Design review of the part built by this model. Coordinates are the model's own, in mm. Face numbers are marked on the shaded views. A direction names the side the tool comes from. Coordinates: 2 decimals unless noted, no trailing zeros. Write each loop counter-clockwise with the first axis right and the second up, starting at its lowest first coordinate (ties: lowest second). Pieces come first, ordered by that corner, then holes. Notation, with made-up numbers: (4, 73) - (62, 73) arc R23 ccw to (62, 105) - close; hole circle Ø7 at (62.5, 37). An arc over 180 degrees is marked (long way). Use a Markdown table: item, result.
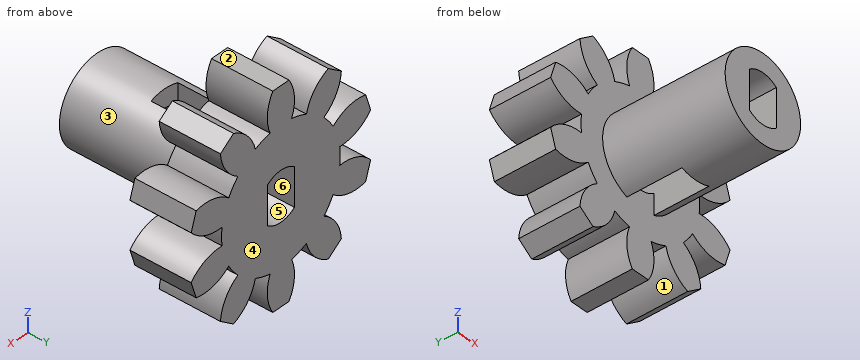
from build123d import *

# Parameters (mm, degrees)
SKETCH_1_R                      = 5.5
EXTRUDE_1_DEPTH                 = 5
EXTRUDE_START                   = -5
EXTRUDE_2_DEPTH                 = 5
SKETCH_3_R                      = 3.5
EXTRUDE_3_DEPTH                 = 10
CUT_EXTRUDE_1_DEPTH             = 20.141619155
CUT_EXTRUDE_2_REACH             = 17.537
SKETCH_5_W                      = 2.5
SKETCH_5_H                      = 4.5
CUT_EXTRUDE_2_DIRECTION_2_REACH = 17.537


with BuildPart() as part:
    # 草图1 → 凸台-拉伸1 (new body)
    with BuildSketch(Plane(origin=(0, 0, 0), x_dir=(1, 0, 0), z_dir=(0, 1, 0))):
        with Locations(Location((0, 0, 0), (0, 0, 270))):
            Circle(SKETCH_1_R)
    extrude(amount=EXTRUDE_1_DEPTH)

    # 草图2 → 凸台-拉伸2 (add)
    with BuildSketch(Plane(origin=(0, 5, 0), x_dir=(-1, 0, 0), z_dir=(0, 1, 0)).offset(EXTRUDE_START)):
        with BuildLine():
            Line((-4.389411899, -7.317483391), (-5.60293739, -6.435805513))
            ThreePointArc((-5.60293739, -6.435805513), (-5.11774735, -4.915167527), (-3.987951794, -3.787643132))
            ThreePointArc((-3.987951794, -3.787643132), (-3.232818888, -4.449593469), (-2.369917805, -4.963213636))
            ThreePointArc((-2.369917805, -4.963213636), (-3.093131201, -6.386137262), (-4.389411899, -7.317483391))
        make_face()
        with BuildLine():
            Line((-7.852217643, -3.339936839), (-8.315743134, -1.913352065))
            ThreePointArc((-8.315743134, -1.913352065), (-7.029407564, -0.968317642), (-5.452641547, -0.720208411))
            ThreePointArc((-5.452641547, -0.720208411), (-5.23081084, -1.699593469), (-4.834607559, -2.622321444))
            ThreePointArc((-4.834607559, -2.622321444), (-6.256073009, -3.34839667), (-7.852217643, -3.339936839))
        make_face()
        with BuildLine():
            Line((-8.315743134, 1.913352065), (-7.852217643, 3.339936839))
            ThreePointArc((-7.852217643, 3.339936839), (-6.256073009, 3.34839667), (-4.834607559, 2.622321444))
            ThreePointArc((-4.834607559, 2.622321444), (-5.23081084, 1.699593469), (-5.452641547, 0.720208411))
            ThreePointArc((-5.452641547, 0.720208411), (-7.029407564, 0.968317642), (-8.315743134, 1.913352065))
        make_face()
        with BuildLine():
            Line((-5.60293739, 6.435805513), (-4.389411899, 7.317483391))
            ThreePointArc((-4.389411899, 7.317483391), (-3.093131201, 6.386137262), (-2.369917805, 4.963213636))
            ThreePointArc((-2.369917805, 4.963213636), (-3.232818888, 4.449593469), (-3.987951794, 3.787643132))
            ThreePointArc((-3.987951794, 3.787643132), (-5.11774735, 4.915167527), (-5.60293739, 6.435805513))
        make_face()
        with BuildLine():
            Line((-0.75, 8.5), (0.75, 8.5))
            ThreePointArc((0.75, 8.5), (1.251281594, 6.984590476), (1, 5.408326913))
            ThreePointArc((1, 5.408326913), (0, 5.5), (-1, 5.408326913))
            ThreePointArc((-1, 5.408326913), (-1.251281594, 6.984590476), (-0.75, 8.5))
        make_face()
        with BuildLine():
            Line((4.389411899, 7.317483391), (5.60293739, 6.435805513))
            ThreePointArc((5.60293739, 6.435805513), (5.11774735, 4.915167527), (3.987951794, 3.787643132))
            ThreePointArc((3.987951794, 3.787643132), (3.232818888, 4.449593469), (2.369917805, 4.963213636))
            ThreePointArc((2.369917805, 4.963213636), (3.093131201, 6.386137262), (4.389411899, 7.317483391))
        make_face()
        with BuildLine():
            Line((0.75, -8.5), (-0.75, -8.5))
            ThreePointArc((-0.75, -8.5), (-1.251281594, -6.984590476), (-1, -5.408326913))
            ThreePointArc((-1, -5.408326913), (0, -5.5), (1, -5.408326913))
            ThreePointArc((1, -5.408326913), (1.251281594, -6.984590476), (0.75, -8.5))
        make_face()
        with BuildLine():
            Line((7.852217643, 3.339936839), (8.315743134, 1.913352065))
            ThreePointArc((8.315743134, 1.913352065), (7.029407564, 0.968317642), (5.452641547, 0.720208411))
            ThreePointArc((5.452641547, 0.720208411), (5.23081084, 1.699593469), (4.834607559, 2.622321444))
            ThreePointArc((4.834607559, 2.622321444), (6.256073009, 3.34839667), (7.852217643, 3.339936839))
        make_face()
        with BuildLine():
            Line((8.315743134, -1.913352065), (7.852217643, -3.339936839))
            ThreePointArc((7.852217643, -3.339936839), (6.256073009, -3.34839667), (4.834607559, -2.622321444))
            ThreePointArc((4.834607559, -2.622321444), (5.23081084, -1.699593469), (5.452641547, -0.720208411))
            ThreePointArc((5.452641547, -0.720208411), (7.029407564, -0.968317642), (8.315743134, -1.913352065))
        make_face()
        with BuildLine():
            Line((5.60293739, -6.435805513), (4.389411899, -7.317483391))
            ThreePointArc((4.389411899, -7.317483391), (3.093131201, -6.386137262), (2.369917805, -4.963213636))
            ThreePointArc((2.369917805, -4.963213636), (3.232818888, -4.449593469), (3.987951794, -3.787643132))
            ThreePointArc((3.987951794, -3.787643132), (5.11774735, -4.915167527), (5.60293739, -6.435805513))
        make_face()
    extrude(amount=EXTRUDE_2_DEPTH)

    # 草图3 → 凸台-拉伸3 (add)
    with BuildSketch(Plane.XZ):
        with Locations(Location((0, 0, 0), (0, 0, 90))):
            Circle(SKETCH_3_R)
    extrude(amount=EXTRUDE_3_DEPTH)

    # 草图4 → 切除-拉伸1 (cut, through all)
    with BuildSketch(Plane(origin=(0, 5, 0), x_dir=(-1, 0, 0), z_dir=(0, 1, 0))):
        with BuildLine():
            Line((1.25, 1.5612495), (1.25, -1.5612495))
            ThreePointArc((1.25, -1.5612495), (0, -2), (-1.25, -1.5612495))
            Line((-1.25, -1.5612495), (-1.25, 1.5612495))
            ThreePointArc((-1.25, 1.5612495), (0, 2), (1.25, 1.5612495))
        make_face()
    extrude(amount=-CUT_EXTRUDE_1_DEPTH, mode=Mode.SUBTRACT)

    # 草图5 → 切除-拉伸2 (cut, up to next)
    with BuildSketch(Plane.XY, mode=Mode.PRIVATE) as cut_extrude_2_sk1:
        with Locations((0, -2.25)):
            Rectangle(SKETCH_5_W, SKETCH_5_H)
    cut_extrude_2_tool1 = extrude(cut_extrude_2_sk1.sketch, amount=-CUT_EXTRUDE_2_REACH, mode=Mode.PRIVATE) & part.part
    add(cut_extrude_2_tool1.solids().sort_by_distance((0, -2.25, 0))[0], mode=Mode.SUBTRACT)

    # 草图5 → 切除-拉伸2 direction 2 (cut, up to next)
    with BuildSketch(Plane.XY, mode=Mode.PRIVATE) as cut_extrude_2_direction_2_sk1:
        with Locations((0, -2.25)):
            Rectangle(SKETCH_5_W, SKETCH_5_H)
    cut_extrude_2_direction_2_tool1 = extrude(cut_extrude_2_direction_2_sk1.sketch, amount=CUT_EXTRUDE_2_DIRECTION_2_REACH, mode=Mode.PRIVATE) & part.part
    add(cut_extrude_2_direction_2_tool1.solids().sort_by_distance((0, -2.25, 0))[0], mode=Mode.SUBTRACT)


solid = part.part
(1) Machinability: for the marked faces 4, 5 and 6, which of the approach directions +Z, -Z, +X, -X, +Y, -Y give a long, thin tool a straight path to every point of the face, cutting with its end or side? Answer none if there is none.
Determined:
| item | result |
|---|---|
| face 4 | +Z, -Z, +X, -X, +Y |
| face 5 | +Y, -Y |
| face 6 | none |
(2) Take a section at D-D on y = -0.25. Write out the cut boundary in (x, z).
Determined:
| item | result |
|---|---|
| outline | (-1.25, -3.27) - (-1.25, 3.27) arc R3.5 ccw to start; (1.25, -3.27) arc R3.5 ccw to (1.25, 3.27) - close |
(3) Take a section at A-A on z = 0. Write out the cut boundary in (x, y).
Determined:
| item | result |
|---|---|
| outline | (-5.5, 0) - (-3.5, 0) - (-3.5, -10) - (-1.25, -10) - (-1.25, 5) - (-5.5, 5) - close; (1.25, -10) - (3.5, -10) - (3.5, 0) - (5.5, 0) - (5.5, 5) - (1.25, 5) - close |
(4) Take a section at B-B on x = 0. Write out the cut boundary in (y, z), and give its area (3 significant figures).
Determined:
| item | result |
|---|---|
| outline | (-10, -3.5) - (-4.5, -3.5) - (-4.5, -2) - (-10, -2) - close; (-10, 2) - (-4.5, 2) - (-4.5, 3.5) - (-10, 3.5) - close; (0, -8.5) - (5, -8.5) - (5, -2) - (0, -2) - close; (0, 2) - (5, 2) - (5, 8.5) - (0, 8.5) - close |
| area | 81.5 mm2 |
(5) For pin 1 (5 mm diameter, centred on y = 1, z = 1, fed in from +X); pin 2 (1 mm diameter, centred on x = 0.5, z = 5, fed in from -Y); pin 3 (5 mm diameter, centred on y = -5, z = 0, fed in from -X); pin 4 (6 mm diameter, centred on y = 0.5, z = -5.5, fed in from +X), all flat-tipped, find the tip position at first contact; note any pin that passes through.
Determined:
| item | result |
|---|---|
| pin 1 | x = 8.32 |
| pin 2 | y = 0 |
| pin 3 | x = -3.5 |
| pin 4 | x = 8.13 |
(6) Take a section at C-C on x = 7.25. Write out the cut boundary in (y, z), and give its area (3 significant figures).
Determined:
| item | result |
|---|---|
| outline | (0, -3.43) - (5, -3.43) - (5, -1.07) - (0, -1.07) - close; (0, 1.07) - (5, 1.07) - (5, 3.43) - (0, 3.43) - close |
| area | 23.6 mm2 |
(7) Draft analysis for pull direction X (two halves, no side actions). For the marked faces 1, 2 and 3, state which applies: +X half, -X half, draft (parallel to the pull), parting line (faces both ways), or undercut.
Determined:
| item | result |
|---|---|
| face 1 | undercut |
| face 2 | draft |
| face 3 | parting line |
(8) For L1, parallel to X at y = 3.5, z = 0.25; L2, parallel to X at y = 2.5, z = 2.75; L3, parallel to Z at x = 4.25, y = 4, list the stretches that pass through material, from the lowest coordinate up. Write a range as from..to.
Determined:
| item | result |
|---|---|
| L1 | -5.49..-1.25, 1.25..5.49 |
| L2 | -8.04..-4.99, -4.76..4.76, 4.99..8.04 |
| L3 | -7.26..-3.96, -3.49..3.49, 3.96..7.26 |
